from build123d import *

# Parameters (mm, degrees)
SKETCH1_W                                           = 66
SKETCH1_H                                           = 29.5
BOSS_EXTRUDE1_DEPTH                                 = 7
SKETCH18_W                                          = 5
SKETCH18_H                                          = 1
BOSS_EXTRUDE3_DEPTH                                 = 3
SKETCH2_W                                           = 64
SKETCH2_H                                           = 27.5
CUT_EXTRUDE1_DEPTH                                  = 1.6
SKETCH19_W                                          = 25.008900438
SKETCH19_H                                          = 27.5
SKETCH19_W_2                                        = 25.033550957
CUT_EXTRUDE3_DEPTH                                  = 10
CSK_FOR_M3_COUNTERSUNK_FLAT_HEAD_SCREW2_D           = 3.4
CSK_FOR_M3_COUNTERSUNK_FLAT_HEAD_SCREW2_CSINK_D     = 6.3
CSK_FOR_M3_COUNTERSUNK_FLAT_HEAD_SCREW2_CSINK_ANGLE = 90


with BuildPart() as part:
    # Sketch1 → Boss-Extrude1 (new body)
    with BuildSketch(Plane(origin=(0, 0, 0), x_dir=(1, 0, 0), z_dir=(0, 1, 0))):
        with Locations((33, -14.75)):
            Rectangle(SKETCH1_W, SKETCH1_H)
    extrude(amount=BOSS_EXTRUDE1_DEPTH)

    # Sketch18 → Boss-Extrude3 (add)
    with BuildSketch(Plane(origin=(0, 7, 0), x_dir=(1, 0, 0), z_dir=(0, 1, 0))):
        with Locations((33, -0.5)):
            Rectangle(SKETCH18_W, SKETCH18_H)
        with Locations((33, -29)):
            Rectangle(SKETCH18_W, SKETCH18_H)
    extrude(amount=BOSS_EXTRUDE3_DEPTH)

    # Sketch2 → Cut-Extrude1 (cut)
    with BuildSketch(Plane(origin=(0, 7, 0), x_dir=(1, 0, 0), z_dir=(0, 1, 0))):
        with Locations((33, -14.75)):
            Rectangle(SKETCH2_W, SKETCH2_H)
    extrude(amount=-CUT_EXTRUDE1_DEPTH, mode=Mode.SUBTRACT)

    # Sketch19 → Cut-Extrude3 (cut)
    with BuildSketch(Plane(origin=(0, 5.4, 0), x_dir=(1, 0, 0), z_dir=(0, 1, 0))):
        with Locations((14.504450219, -14.75)):
            Rectangle(SKETCH19_W, SKETCH19_H)
        with Locations((51.483224522, -14.75)):
            Rectangle(SKETCH19_W_2, SKETCH19_H)
    extrude(amount=-CUT_EXTRUDE3_DEPTH, mode=Mode.SUBTRACT)

    # CSK for M3 Countersunk Flat Head Screw2 (through all)
    with Locations(Plane(origin=(32.966449043, 5.4, 7.875), x_dir=(0, 0, 1), z_dir=(0, 1, 0))):
        with Locations((0, 0), (15.515633601, 0.042451395)):
            CounterSinkHole(CSK_FOR_M3_COUNTERSUNK_FLAT_HEAD_SCREW2_D / 2, CSK_FOR_M3_COUNTERSUNK_FLAT_HEAD_SCREW2_CSINK_D / 2, counter_sink_angle=CSK_FOR_M3_COUNTERSUNK_FLAT_HEAD_SCREW2_CSINK_ANGLE)


solid = part.part
Design review of the part built by this model. Coordinates are the model's own, in mm. A direction names the side the tool comes from. Round coordinates to 2 decimals unless told otherwise and drop trailing zeros. Loops run counter-clockwise (first coordinate to the right, second up) from the corner with the lowest first, then second, coordinate; pieces in that order, holes last. Notation, with made-up numbers: (10.25, 29.5) - (34.25, 29.5) arc R17 ccw to (34.25, 41.5) - close; hole circle Ø7 at (15, 88.5). An arc over 180 degrees is marked (long way). One line per question, with ' | ' between items.
1. For faces 5 (the face through (65, 6, 15)), 6 (the face through (0.5, 7, 14.7)), 7 (the face through (64, 3, 15)), list the 3-axis set-ups (+Z, -Z, +X, -X, +Y, -Y) from which the entire face can be reached by the end or side of a thin tool; tool diameter is ignored.
Results are:
face 5: +Y | face 6: +Z, -Z, -X, +Y | face 7: +Y, -Y
2. We need section A-A, the plane x = 54.5. State the section outline as (y, z) points.
Results are:
outline: (0, 0) - (7, 0) - (7, 1) - (0, 1) - close; (0, 28.5) - (7, 28.5) - (7, 29.5) - (0, 29.5) - close
3. We need section D-D, the plane z = 23.5. State how many separate pieces and enclosed holes the cut face has, and give its area (3 significant figures).
Results are:
separate pieces: 4 | enclosed holes: 0 | area: 68.9 mm²
4. For L1, parallel to X at y = 4.5, z = 15; L2, parallel to Z at x = 24.5, y = 5.5; L3, parallel to X at y = 4.5, z = 8.5 (3 decimals), list the stretches that pass through material, from the lowest coordinate up. Write a range as [from, to].
Results are:
L1: x = [0, 2], [27.01, 38.97], [64, 66] | L2: z = [0, 1], [28.5, 29.5] | L3: x = [0, 2], [27.009, 30.805], [35.128, 38.966], [64, 66]
5. We need section C-C, the plane y = 6. State the section outline as (x, z) points.
Results are:
outline: (0, 0) - (66, 0) - (66, 29.5) - (0, 29.5) - close; hole (1, 1) - (65, 1) - (65, 28.5) - (1, 28.5) - close
6. Draft analysis for pull direction Z (two halves, no side actions). For faces 1 (the face through (33, 4, 29.5)), 2 (the face through (33, 4, 0)), 3 (the face through (0, 3, 15)), 4 (the face through (2, 3, 15)), state which applies: released by +Z, released by -Z, zero draft, split by the parting line, or undercut.
Results are:
face 1: released by +Z | face 2: released by -Z | face 3: zero draft | face 4: undercut
7. We need section B-B, the plane z = 13.75. State the section outline as (x, y) points, and give its area (3 significant figures).
Results are:
outline: (0, 0) - (2, 0) - (2, 5.4) - (1, 5.4) - (1, 7) - (0, 7) - close; (27.01, 0) - (38.97, 0) - (38.97, 5.4) - (27.01, 5.4) - close; (64, 0) - (66, 0) - (66, 7) - (65, 7) - (65, 5.4) - (64, 5.4) - close | area: 89.4 mm²
8. Clearance check with flat-ended pins moving along their axes: P1, Ø1.6, axis at y = 2.5, z = 16.5, coming from the -X side; P2, Ø2.5, axis at x = 33.01, z = 23.39, coming from the -Y side; P3, Ø0.5, axis at x = 64.5, z = 15.5, coming from the +Y side; P4, Ø1.1, axis at y = 8.5, z = 0.5, coming from the +X side. State where each tip first meets the part, or that it passes through.
Results are:
P1: stops at x = 0 | P2: passes through | P3: stops at y = 5.4 | P4: stops at x = 35.5
